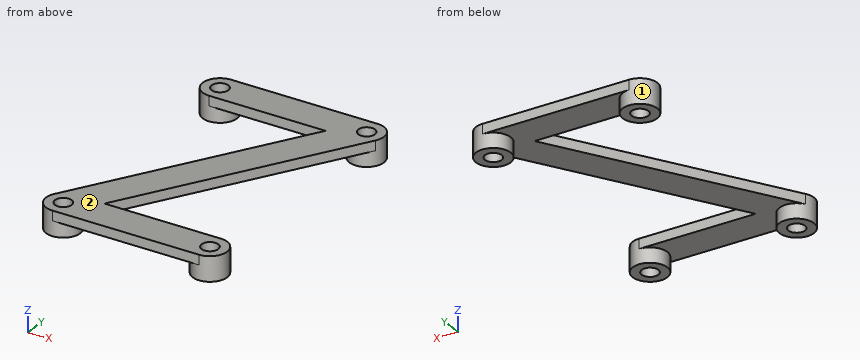
```python
from build123d import *

# Parameters (mm, degrees)
EXTRUDE_944_DEPTH  = 2
SKETCH_1_3_R       = 3.5
SKETCH_1_3_R_2     = 1.7
EXTRUDE_1016_DEPTH = 5


with BuildPart() as part:
    # Эскиз1 → Extrude 944 (new body)
    with BuildSketch(Plane.XY):
        with BuildLine():
            Line((15, 28.5), (-15, 28.5))
            ThreePointArc((-15, 28.5), (-12.525126266, 27.474873734), (-11.5, 25))
            ThreePointArc((-11.5, 25), (-12.525126266, 22.525126266), (-15, 21.5))
            Line((-15, 21.5), (8.818333674, 21.5))
            Line((8.818333674, 21.5), (-18.00122524, -23.199264856))
            ThreePointArc((-18.00122524, -23.199264856), (-14.065732463, -21.626997751), (-11.5, -25))
            ThreePointArc((-11.5, -25), (-12.525126266, -27.474873734), (-15, -28.5))
            Line((-15, -28.5), (15, -28.5))
            ThreePointArc((15, -28.5), (11.5, -25), (15, -21.5))
            Line((15, -21.5), (-8.818333674, -21.5))
            Line((-8.818333674, -21.5), (18.00122524, 23.199264856))
            ThreePointArc((18.00122524, 23.199264856), (11.954300326, 23.275554148), (15, 28.5))
        make_face()
    extrude(amount=-EXTRUDE_944_DEPTH)

    # Эскиз1<3> → Extrude 1016 (add)
    # profile 1 of 4: a face of its own
    with BuildSketch(Plane.XY):
        with Locations((15, 25)):
            Circle(SKETCH_1_3_R)
        with Locations((15, 25)):
            Circle(SKETCH_1_3_R_2, mode=Mode.SUBTRACT)
    # profile 2 of 4: a face of its own
    with BuildSketch(Plane.XY):
        with Locations((15, -25)):
            Circle(SKETCH_1_3_R)
        with Locations((15, -25)):
            Circle(SKETCH_1_3_R_2, mode=Mode.SUBTRACT)
    # profile 3 of 4: a face of its own
    with BuildSketch(Plane.XY):
        with Locations((-15, -25)):
            Circle(SKETCH_1_3_R)
        with Locations((-15, -25)):
            Circle(SKETCH_1_3_R_2, mode=Mode.SUBTRACT)
    # profile 4 of 4: a face of its own
    with BuildSketch(Plane.XY):
        with Locations((-15, 25)):
            Circle(SKETCH_1_3_R)
        with Locations((-15, 25)):
            Circle(SKETCH_1_3_R_2, mode=Mode.SUBTRACT)
    extrude(amount=-EXTRUDE_1016_DEPTH)


solid = part.part
```
The model under review builds one solid part; all positions refer to its coordinate system, in mm. Face numbers are marked on the shaded views. Round coordinates to 2 decimals unless told otherwise and drop trailing zeros. Loops run counter-clockwise (first coordinate to the right, second up) from the corner with the lowest first, then second, coordinate; pieces in that order, holes last. Notation, with made-up numbers: (26.25, -23.5) - (63.25, -23.5) arc R32 cw to (63.25, 6.5) - close; hole circle Ø3 at (39.5, 10.5). An arc over 180 degrees is marked (long way). Use a Markdown table: item, result. Add a question column.
Q1. Add section D-D (x = 7). State the section outline as (y, z) points.
Q2. Add section B-B (y = -25). State the section outline as (x, z) points, plus the area to 3 significant figures.
Q3. Add section C-C (x = -14). State the section outline as (y, z) points, plus the area to 3 significant figures.
Q4. Add section A-A (z = -3.1). State the section outline as (x, y) points, plus the area to 3 significant figures.
Q5. For probe 1 along Y at (x, z) = (-15, -2.85); probe 2 along Y at (x, z) = (-13.5, -4.1); probe 3 along Z at (x, y) = (1, 23.5), list the stretches that pass through material, from the lowest coordinate up.
Q6. The part is to be moulded in two halves that separate along X. For the marked faces 1 and 2, say which applies: pulls with the +X half, pulls with the -X half, needs draft (parallel to the pull), parting line crosses it, or undercut.
Worked answers:
| question | item | result |
|---|---|---|
| 1 | outline | (-28.5, -2) - (-21.5, -2) - (-21.5, 0) - (-28.5, 0) - close; (4.86, -2) - (18.47, -2) - (18.47, 0) - (4.86, 0) - close; (21.5, -2) - (28.5, -2) - (28.5, 0) - (21.5, 0) - close |
| 2 | outline | (-18.5, -5) - (-16.7, -5) - (-16.7, 0) - (-18.5, 0) - close; (-13.3, -5) - (-11.5, -5) - (-11.5, -2) - (11.5, -2) - (11.5, -5) - (13.3, -5) - (13.3, 0) - (-13.3, 0) - close; (16.7, -5) - (18.5, -5) - (18.5, 0) - (16.7, 0) - close |
| 2 | area | 82.0 mm² |
| 3 | outline | (-28.5, -2) - (-28.35, -2) - (-28.35, -5) - (-26.37, -5) - (-26.37, 0) - (-28.5, 0) - close; (-23.63, -5) - (-21.65, -5) - (-21.65, -2) - (-16.53, -2) - (-16.53, 0) - (-23.63, 0) - close; (21.5, -2) - (21.65, -2) - (21.65, -5) - (23.63, -5) - (23.63, 0) - (21.5, 0) - close; (26.37, -5) - (28.35, -5) - (28.35, -2) - (28.5, -2) - (28.5, 0) - (26.37, 0) - close |
| 3 | area | 50.7 mm² |
| 4 | outline | circle Ø7 at (-15, -25); circle Ø7 at (-15, 25); circle Ø7 at (15, -25); circle Ø7 at (15, 25); hole circle Ø3.4 at (-15, -25); hole circle Ø3.4 at (-15, 25); hole circle Ø3.4 at (15, -25); hole circle Ø3.4 at (15, 25) |
| 4 | area | 118 mm² |
| 5 | probe 1 | -28.5 to -26.7, -23.3 to -21.5, 21.5 to 23.3, 26.7 to 28.5 |
| 5 | probe 2 | -28.16 to -25.8, -24.2 to -21.84, 21.84 to 24.2, 25.8 to 28.16 |
| 5 | probe 3 | -2 to 0 |
| 6 | face 1 | undercut |
| 6 | face 2 | needs draft |
